Check sheet for the modelled part. Datum: model origin and axes. Units: mm. A direction names the side the tool comes from. Round coordinates to 2 decimals unless told otherwise and drop trailing zeros. Loops run counter-clockwise (first coordinate to the right, second up) from the corner with the lowest first, then second, coordinate; pieces in that order, holes last. Notation, with made-up numbers: M 31,-29 L 40,-29 A12 ccw 40,-25 Z; hole C 53,68 d8. An arc over 180 degrees is marked long. One line per question, with ' | ' between items. Start each with the question number.
(1) Tool access check on faces 4 (the face through (-2.343, -17.847, 2.465)), 5 (the face through (22.5, 0, 10)). Record the directions out of +Z, -Z, +X, -X, +Y, -Y that give a thin tool (end or side, any length) a straight path to the whole face; none if there is none.
(2) Section check D-D (y = 17). Record the boundary of the cut face in (x, z).
(3) Go/stop test with flat-tipped pins: P1, Ø10, axis at x = -8, y = -3.5, coming from the -Z side; P2, Ø16, axis at x = 0, y = 0, coming from the -Z side. Record where each tip stops, or that it passes through.
(4) Draft check along X on faces 1 (the face through (-22.5, 0, 10)), 2 (the face through (-15.3, 10.3, 0)), 3 (the face through (-2.17, 9.76, 10.92)). Enter one of: +X half, -X half, draft (parallel to the pull), parting line (faces both ways), or undercut.
(5) Section check A-A (y = 0). Record the boundary of the cut face in (x, z).
(6) Thickness scan on probe 1 along Y at (x, z) = (0, 1.1); probe 2 along X at (y, z) = (0, 13). Record the ranges inside material, lowest first. Write a range as [from, to].
(7) Section check B-B (z = 15). Record the boundary of the cut face in (x, y), and give its area (3 significant figures).
```python
from build123d import *

# Parameters (mm, degrees)
F0_W     = 45
F0_H     = 45
F1_DEPTH = 20
F2_R     = 10
F4_DEPTH = 17
F3_R     = 18
F3_R_2   = 10
F5_DEPTH = 5


with BuildPart() as f1:
    # F0 (on Top) → F1 (new body)
    with BuildSketch(Plane.XY):
        Rectangle(F0_W, F0_H)
    extrude(amount=F1_DEPTH)

    # F2 (on face) → F4 (cut)
    with BuildSketch(Plane(origin=(0, 0, 0), x_dir=(1, 0, 0), z_dir=(0, 0, -1))):
        Circle(F2_R)
    extrude(amount=-F4_DEPTH, mode=Mode.SUBTRACT)

    # F3 (on face) → F5 (cut)
    with BuildSketch(Plane(origin=(0, 0, 0), x_dir=(1, 0, 0), z_dir=(0, 0, -1))):
        Circle(F3_R)
        Circle(F3_R_2, mode=Mode.SUBTRACT)
    extrude(amount=-F5_DEPTH, mode=Mode.SUBTRACT)


solid = f1.part
```
The answers:
1) face 4: -Z | face 5: +Z, -Z, +X, +Y, -Y
2) outline: M -22.5,0 L -5.92,0 L -5.92,5 L 5.92,5 L 5.92,0 L 22.5,0 L 22.5,20 L -22.5,20 Z
3) P1: z = 5 | P2: z = 17
4) face 1: -X half | face 2: draft | face 3: undercut
5) outline: M -22.5,0 L -18,0 L -18,5 L -10,5 L -10,17 L 10,17 L 10,5 L 18,5 L 18,0 L 22.5,0 L 22.5,20 L -22.5,20 Z
6) probe 1: [-22.5, -18], [18, 22.5] | probe 2: [-22.5, -10], [10, 22.5]
7) outline: M -22.5,-22.5 L 22.5,-22.5 L 22.5,22.5 L -22.5,22.5 Z; hole C 0,0 d20 | area: 1,710 mm²
